from build123d import *

# Parameters (mm, degrees)
SKETCH_1_R          = 10
EXTRUDE_1_DEPTH     = 270
SKETCH_2_OUTSIDE_W  = 76.296
SKETCH_2_OUTSIDE_H  = 76.296
SKETCH_2_OUTSIDE_R  = 8
CUT_EXTRUDE_2_DEPTH = 56
FILLET_1_R          = 1.6
CHAMFER_1_SIZE      = 1


with BuildPart() as part:
    # Эскиз1 → Вытянуть1 (new body)
    with BuildSketch(Plane(origin=(0, 0, 0), x_dir=(1, 0, 0), z_dir=(0, 1, 0))):
        Circle(SKETCH_1_R)
    extrude(amount=EXTRUDE_1_DEPTH)

    # Эскиз2 outside → Вытянуть2 (cut)
    with BuildSketch(Plane(origin=(0, 270, 0), x_dir=(1, 0, 0), z_dir=(0, 1, 0))):
        Rectangle(SKETCH_2_OUTSIDE_W, SKETCH_2_OUTSIDE_H)
        Circle(SKETCH_2_OUTSIDE_R, mode=Mode.SUBTRACT)
    extrude(amount=-CUT_EXTRUDE_2_DEPTH, mode=Mode.SUBTRACT)

    # Скругление1
    fillet_1_edges = [part.edges().sort_by_distance(p)[0] for p in [
        (-8, 214, 0),
    ]]
    fillet(fillet_1_edges, radius=FILLET_1_R)

    # Фаска1
    chamfer_1_edges = [part.edges().sort_by_distance(p)[0] for p in [
        (-8, 270, 0),
        (-10, 0, 0),
    ]]
    chamfer(chamfer_1_edges, length=CHAMFER_1_SIZE)


solid = part.part
Here's how the part is built. I have some questions about the finished solid (model axes, mm). A direction names the side the tool comes from. Give positions to 0.01 mm unless a question says otherwise; leave off trailing zeros. Order: outer loops, then holes, each group sorted by start corner. A loop starts at its lowest first (then second) coordinate and runs counter-clockwise, first axis right, second up. Notation, with made-up numbers: (74.25, 41) -> (130.25, 41) arc R18 ccw to (130.25, 75) -> close; hole circle Ø10 at (43.5, -5.75). An arc over 180 degrees is marked (long way). Use a Markdown table: item, result. Add a question column.
Item 1: Will these pins go through, and if not, where does the flat tip stop? pin 1 (5 mm diameter, centred on x = -6.5, y = 160, fed in from +Z); pin 2 (10 mm diameter, centred on x = -5.5, y = 91.5, fed in from +Z); pin 3 (12 mm diameter, centred on y = 239.5, z = 8, fed in from -X).
Item 2: I need wall thicknesses on line 1 (X direction, y = 197.5, z = 0.75); line 2 (Z direction, x = -6, y = 100.5); line 3 (Y direction, x = 5.75, z = -5). Which ranges of each line are inside material? Lowest first, please.
Item 3: Imagine slicing it at C-C on y = 232. Please give me the cut outline in (x, z), plus the area to 3 significant figures.
Item 4: Imagine slicing it at B-B on z = 0. Please give me the cut outline in (x, y), plus the area to 3 significant figures.
Item 5: Imagine slicing it at A-A on x = 0. Please give me the cut outline in (y, z).
Item 6: Imagine slicing it at D-D on y = 20. Please give me the cut outline in (x, z), plus the area to 3 significant figures.
Item 7: For faces 1 (the face through (0, 270, 0)), 2 (the face through (-1.73, 242.67, 7.81)), which set-ups out of +Z, -Z, +X, -X, +Y, -Y let a thin tool reach every point of the face, with its end or its side?
Data:
| question | item | result |
|---|---|---|
| 1 | pin 1 | stops at z = 9.17 |
| 1 | pin 2 | stops at z = 9.99 |
| 1 | pin 3 | stops at x = -7.75 |
| 2 | line 1 | x = -9.97 to 9.97 |
| 2 | line 2 | z = -8 to 8 |
| 2 | line 3 | y = 0 to 269.38 |
| 3 | outline | circle Ø16 at (0, 0) |
| 3 | area | 201 mm² |
| 4 | outline | (-10, 1) -> (-9, 0) -> (9, 0) -> (10, 1) -> (10, 214) -> (9.6, 214) arc R1.6 cw to (8, 215.6) -> (8, 269) -> (7, 270) -> (-7, 270) -> (-8, 269) -> (-8, 215.6) arc R1.6 cw to (-9.6, 214) -> (-10, 214) -> close |
| 4 | area | 5,180 mm² |
| 5 | outline | (0, -9) -> (1, -10) -> (214, -10) -> (214, -9.6) arc R1.6 cw to (215.6, -8) -> (269, -8) -> (270, -7) -> (270, 7) -> (269, 8) -> (215.6, 8) arc R1.6 cw to (214, 9.6) -> (214, 10) -> (1, 10) -> (0, 9) -> close |
| 6 | outline | circle Ø20 at (0, 0) |
| 6 | area | 314 mm² |
| 7 | face 1 | +Z, -Z, +X, -X, +Y |
| 7 | face 2 | +Y |
